CAD build for the part. Positions are in the model's coordinates, mm. A direction names the side the tool comes from. Coordinates: 2 decimals unless noted, no trailing zeros. Write each loop counter-clockwise with the first axis right and the second up, starting at its lowest first coordinate (ties: lowest second). Pieces come first, ordered by that corner, then holes. Notation, with made-up numbers: (-23.75, -12.75) - (6.25, -12.75) arc R24 ccw to (6.25, 7.25) - close; hole circle Ø8 at (-31.75, 69.5). An arc over 180 degrees is marked (long way). Answer in a Markdown table with one row per item. Add a question column.
Q1. Band-saw the part on C-C (y = 4). List the corners of the cut face in (x, z).
Q2. Drill centre lines: line 1 along Y through (x, z) = (64, 0.7); line 2 along Y through (x, z) = (8, 1.55); line 3 along X through (y, z) = (-1.75, 0.85). Where is each one in solid material? Low to high. Write a range as from..to.
Q3. Band-saw the part on B-B (z = 0.5). List the corners of the cut face in (x, y).
Q4. Two-plate mould, pull along X, no slides. Class faces 1 (the cylindrical face through (72.9, 13, 1)), 2 (the cylindrical face through (-7, 0, 1)), 3 (the cylindrical face through (62.92, -0.88, 1.01)), 4 (the cylindrical face through (14.4, -1.2, 1)): +X half, -X half, draft (parallel to the pull), parting line (faces both ways), or undercut.
Q5. 3-axis set-ups, long thin cutter, end or side, ignore diameter. For faces 5 (the cylindrical face through (6, 0, 1)), 6 (the flat face through (16, 7, 1)): which of +Z, -Z, +X, -X, +Y, -Y reach the whole face in a straight line?
Q6. Band-saw the part on A-A (x = 64). List the corners of the cut face in (y, z), and give its area (3 significant figures).
Q7. Pin check, flat tips, straight feed: pin 1 (1 mm diameter, centred on y = -1.5, z = 0.5, fed in from -X); pin 2 (1 mm diameter, centred on y = -4.5, z = 1.5, fed in from +X). Stop position of each tip, or through.
Q8. Band-saw the part on D-D (y = 0.75). List the corners of the cut face in (x, z).
```python
from build123d import *

# Parameters (mm, degrees)
BOSS_EXTRUDE1_DEPTH = 2
SKETCH2_R           = 2
CUT_EXTRUDE1_DEPTH  = 2
SKETCH3_R           = 5
CUT_EXTRUDE2_DEPTH  = 2


with BuildPart() as part:
    # Sketch1 → Boss-Extrude1 (new body)
    with BuildSketch(Plane.XY):
        with BuildLine():
            Line((0, 7), (33, 7))
            ThreePointArc((33, 7), (44.66919932, 8.739971416), (55.323194976, 13.808510638))
            ThreePointArc((55.323194976, 13.808510638), (57.187644216, 14.695505002), (59.229754097, 15))
            Line((59.229754097, 15), (68, 15))
            ThreePointArc((68, 15), (72.949747468, 12.949747468), (75, 8))
            Line((75, 8), (75, 0))
            ThreePointArc((75, 0), (72.949747468, -4.949747468), (68, -7))
            Line((68, -7), (0, -7))
            ThreePointArc((0, -7), (-7, 0), (0, 7))
        make_face()
    extrude(amount=BOSS_EXTRUDE1_DEPTH)

    # Sketch2 → Cut-Extrude1 (cut)
    with BuildSketch(Plane.XY.offset(2)):
        Circle(SKETCH2_R)
        with Locations((8, 0)):
            Circle(SKETCH2_R)
        with Locations((16, 0)):
            Circle(SKETCH2_R)
    extrude(amount=-CUT_EXTRUDE1_DEPTH, mode=Mode.SUBTRACT)

    # Sketch3 → Cut-Extrude2 (cut)
    with BuildSketch(Plane.XY.offset(2)):
        with Locations((64, 4)):
            Circle(SKETCH3_R)
    extrude(amount=-CUT_EXTRUDE2_DEPTH, mode=Mode.SUBTRACT)


solid = part.part
```
Checked values:
| question | item | result |
|---|---|---|
| 1 | outline | (-5.74, 0) - (59, 0) - (59, 2) - (-5.74, 2) - close; (69, 0) - (75, 0) - (75, 2) - (69, 2) - close |
| 2 | line 1 | y = -7..-1, 9..15 |
| 2 | line 2 | y = -7..-2, 2..7 |
| 2 | line 3 | x = -6.78..-0.97, 0.97..7.03, 8.97..15.03, 16.97..74.78 |
| 3 | outline | (0, -7) - (68, -7) arc R7 ccw to (75, 0) - (75, 8) arc R7 ccw to (68, 15) - (59.23, 15) arc R7 ccw to (55.32, 13.81) arc R40 cw to (33, 7) - (0, 7) arc R7 ccw to start; hole circle Ø4 at (0, 0); hole circle Ø4 at (8, 0); hole circle Ø4 at (16, 0); hole circle Ø10 at (64, 4) |
| 4 | face 1 | +X half |
| 4 | face 2 | -X half |
| 4 | face 3 | undercut |
| 4 | face 4 | undercut |
| 5 | face 5 | +Z, -Z |
| 5 | face 6 | +Z, -Z, -X, +Y |
| 6 | outline | (-7, 0) - (-1, 0) - (-1, 2) - (-7, 2) - close; (9, 0) - (15, 0) - (15, 2) - (9, 2) - close |
| 6 | area | 24.0 mm² |
| 7 | pin 1 | stops at x = -6.93 |
| 7 | pin 2 | stops at x = 73.74 |
| 8 | outline | (-6.96, 0) - (-1.85, 0) - (-1.85, 2) - (-6.96, 2) - close; (1.85, 0) - (6.15, 0) - (6.15, 2) - (1.85, 2) - close; (9.85, 0) - (14.15, 0) - (14.15, 2) - (9.85, 2) - close; (17.85, 0) - (60.2, 0) - (60.2, 2) - (17.85, 2) - close; (67.8, 0) - (75, 0) - (75, 2) - (67.8, 2) - close |
